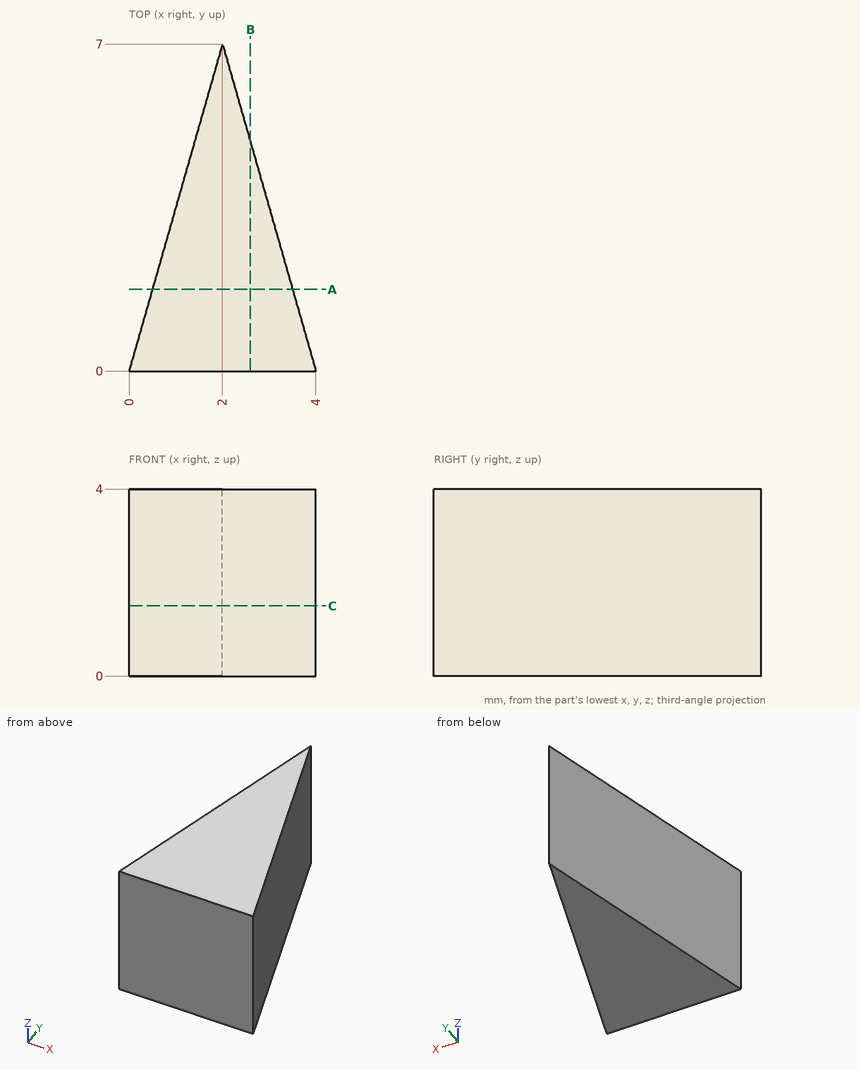
Job drawing, mm, ordinate dimensions from the low corner. One solid piece. Give positions to 0.01 mm unless a question says otherwise; leave off trailing zeros. Write each loop counter-clockwise with the first axis right and the second up, starting at its lowest first coordinate (ties: lowest second). Pieces come first, ordered by that corner, then holes. Notation, with made-up numbers: M 10,-31.75 L 42,-31.75 A35 cw 42,7.25 Z; hole C 50,24.5 d4. An arc over 180 degrees is marked long. Put each result on its own line as item: value. Start each with the question number.
(1) Flat gauge pins, fed straight in: pin 1 Ø2 at (y, z) = (2, 3.5) entering from -X; pin 2 Ø1 at (y, z) = (4, 1.5) entering from +X. Where does each tip first touch, or does it go through?
(2) Band-saw the part on C-C, the plane z = 1.5. Write the cut outline in (x, y).
(3) Band-saw the part on B-B, the plane x = 2.6. Write the cut outline in (y, z), and give its area (3 significant figures).
(4) Band-saw the part on A-A, the plane y = 1.75. Write the cut outline in (x, z).
(5) Probe L1, parallel to X at y = 1, z = 3.8; L2, parallel to X at y = 5.75, z = 3.6. List the from-to ranges inside material, lowest first.
Response values:
1. pin 1: stops at x = 0.29
1. pin 2: stops at x = 3
2. outline: M 0,0 L 4,0 L 2,7 Z
3. outline: M 0,0 L 4.9,0 L 4.9,4 L 0,4 Z
3. area: 19.6 mm2
4. outline: M 0.5,0 L 3.5,0 L 3.5,4 L 0.5,4 Z
5. L1: x = 0.29 to 3.71
5. L2: x = 1.64 to 2.36
